Source: CAD feature listing. Evaluate the final solid. Frame: model axes, mm. Face numbers are marked on the shaded views. A direction names the side the tool comes from. Give positions to 0.01 mm unless a question says otherwise; leave off trailing zeros. Loops run counter-clockwise (first coordinate to the right, second up) from the corner with the lowest first, then second, coordinate; pieces in that order, holes last. Notation, with made-up numbers: M -28.75,67.25 L 3.25,67.25 A24 ccw 3.25,94.25 Z; hole C 76,86.5 d8. An arc over 180 degrees is marked long. Put each result on its own line as item: value.
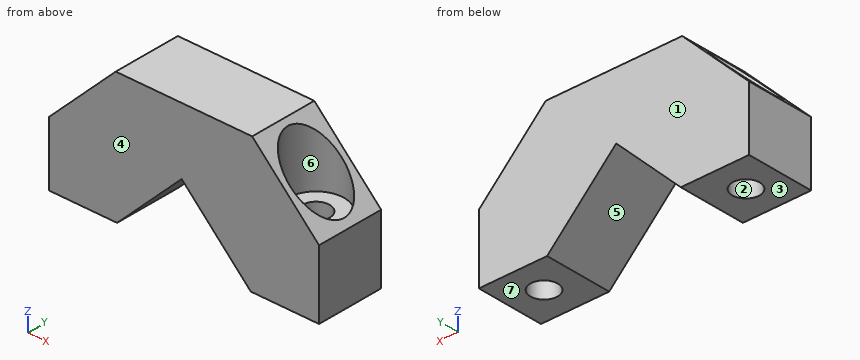
from build123d import *

# Parameters (mm, degrees)
BOSS_EXTRUDE1_DEPTH = 12.7
CUT_EXTRUDE3_START  = 0.848528
SKETCH3_R           = 2.54
CUT_EXTRUDE3_DEPTH  = 12.7
SKETCH4_R           = 5.25
CUT_EXTRUDE4_DEPTH  = 12.7


with BuildPart() as part:
    # Sketch2 → Boss-Extrude1 (new body)
    with BuildSketch(Plane(origin=(0, 0, 0), x_dir=(1, 0, 0), z_dir=(0, 1, 0))):
        Polygon((-23.425952314, 11.801132082), (-11.405137034, -0.219683198), (1.464206384, 12.649660219), (14.164206384, 12.649660219), (14.164206384, -0.050339781), (1.719127035, -12.495419129), (-23.680872965, -12.495419129), (-36.125952314, -0.050339781), (-36.125952314, 11.801132082), align=None)
    extrude(amount=BOSS_EXTRUDE1_DEPTH)

    # Sketch3 → Cut-Extrude3 (cut)
    with BuildSketch(Plane(origin=(0, 0, -11.801132082), x_dir=(-1, 0, 0), z_dir=(0, 0, -1)).offset(CUT_EXTRUDE3_START)):
        with Locations(Location((-7.814206384, 6.35, 0), (0, 0, 180))):
            Circle(SKETCH3_R)
        with Locations(Location((29.775952314, 6.35, 0), (0, 0, 180))):
            Circle(SKETCH3_R)
    extrude(amount=-CUT_EXTRUDE3_DEPTH, mode=Mode.SUBTRACT)

    # Sketch4 → Cut-Extrude4 (cut)
    with BuildSketch(Plane(origin=(0, 0, 0.050339781), x_dir=(-1, 0, 0), z_dir=(0, 0, -1))):
        with Locations((-7.814206384, 6.35)):
            Circle(SKETCH4_R)
        with Locations((29.775952314, 6.35)):
            Circle(SKETCH4_R)
    extrude(amount=-CUT_EXTRUDE4_DEPTH, mode=Mode.SUBTRACT)


solid = part.part
1. Contact query for flat-ended pins moving along their axis: P1, Ø1, axis at x = 1, z = 9, coming from the -Y side; P2, Ø6.5, axis at x = 7.81, y = 6.35, coming from the +Z side; P3, Ø4, axis at y = 10, z = 8, coming from the +X side; P4, Ø4, axis at y = 3, z = 7.5, coming from the -X side. Output: stop coordinate, or through.
Found:
P1: y = 0
P2: z = 0.05
P3: x = 7.43
P4: x = -29.35
2. Section query C-C (z = -10.5). Output: boundary loops of the cut face in (x, y), plus the area to 3 significant figures.
Found:
outline: M -36.13,0 L -22.12,0 L -22.12,12.7 L -36.13,12.7 Z; M -0.69,0 L 14.16,0 L 14.16,12.7 L -0.69,12.7 Z; hole C -29.78,6.35 d5.08; hole C 7.81,6.35 d5.08
area: 326 mm^2
3. Access query for the marked faces 5, 6 and 7. Directions: +Z, -Z, +X, -X, +Y, -Y. A direction counts if a zero-diameter tool reaches every point of the face in a straight line with its end or side. Return the directions, or none.
Found:
face 5: -Z, +Y, -Y
face 6: +Z
face 7: -Z, +X, -X, +Y, -Y
4. Section query D-D (y = 10.75). Output: boundary loops of the cut face in (x, z).
Found:
outline: M -36.13,-11.8 L -23.43,-11.8 L -11.41,0.22 L 1.46,-12.65 L 14.16,-12.65 L 14.16,0.05 L 10.68,3.54 L 10.68,0.05 L 4.95,0.05 L 4.95,9.26 L 1.72,12.5 L -23.68,12.5 L -26.91,9.26 L -26.91,0.05 L -32.64,0.05 L -32.64,3.54 L -36.13,0.05 Z
5. Section query A-A (z = -6.75). Output: boundary loops of the cut face in (x, y).
Found:
outline: M -36.13,0 L -18.37,0 L -18.37,12.7 L -36.13,12.7 Z; M -4.44,0 L 14.16,0 L 14.16,12.7 L -4.44,12.7 Z; hole C -29.78,6.35 d5.08; hole C 7.81,6.35 d5.08
6. Section query B-B (y = 6.35). Output: boundary loops of the cut face in (x, z), plus the area to 3 significant figures.
Found:
outline: M -36.13,-11.8 L -32.32,-11.8 L -32.32,0.05 L -35.03,0.05 L -35.03,1.15 L -36.13,0.05 Z; M -27.24,-11.8 L -23.43,-11.8 L -11.41,0.22 L 1.46,-12.65 L 5.27,-12.65 L 5.27,0.05 L 2.56,0.05 L 2.56,11.65 L 1.72,12.5 L -23.68,12.5 L -24.53,11.65 L -24.53,0.05 L -27.24,0.05 Z; M 10.35,-12.65 L 14.16,-12.65 L 14.16,0.05 L 13.06,1.15 L 13.06,0.05 L 10.35,0.05 Z
area: 676 mm^2
7. Draft query along Y for the marked faces 1, 2, 3 and 4. Return one class per face: pulls with the +Y half, pulls with the -Y half, needs draft (parallel to the pull), parting line crosses it, or undercut.
Found:
face 1: pulls with the +Y half
face 2: undercut
face 3: needs draft
face 4: pulls with the -Y half
8. Material intervals for line 1 (X direction, y = 8.5, z = -1.75); line 2 (X direction, y = 8, z = 0.25); line 3 (X direction, y = 8.5, z = -2.5), sorted ascending. Write a range as from..to.
Found:
line 1: -36.13..-31.13, -28.42..-13.37, -9.44..6.46, 9.17..14.16
line 2: -35.93..-34.76, -24.79..2.83, 12.8..13.96
line 3: -36.13..-31.13, -28.42..-14.12, -8.69..6.46, 9.17..14.16
